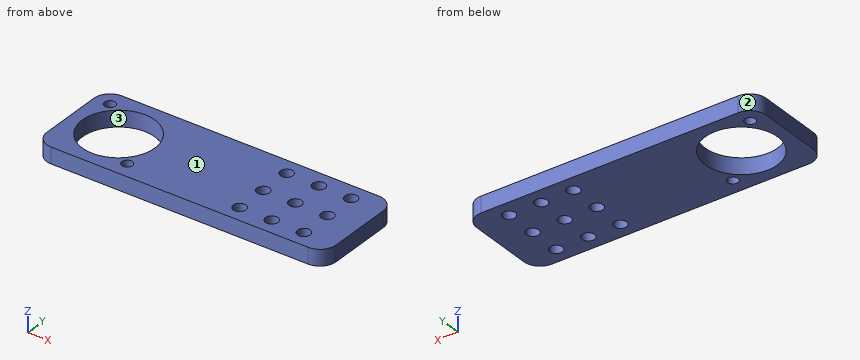
from build123d import *

# Parameters (mm, degrees)
SKETCH1_R           = 14.3002
SKETCH1_R_2         = 2.0828
SKETCH1_R_3         = 2.4892
BOSS_EXTRUDE1_DEPTH = 6.35


with BuildPart() as part:
    # Sketch1 → Boss-Extrude1 (new body)
    with BuildSketch(Plane.XY):
        with BuildLine():
            Line((114.3, -12.7), (114.3, 12.7))
            ThreePointArc((114.3, 12.7), (112.440128061, 17.190128061), (107.95, 19.05))
            Line((107.95, 19.05), (6.35, 19.05))
            ThreePointArc((6.35, 19.05), (1.859871939, 17.190128061), (0, 12.7))
            Line((0, 12.7), (0, -12.7))
            ThreePointArc((0, -12.7), (1.859871939, -17.190128061), (6.35, -19.05))
            Line((6.35, -19.05), (107.95, -19.05))
            ThreePointArc((107.95, -19.05), (112.440128061, -17.190128061), (114.3, -12.7))
        make_face()
        with Locations((19.05, 0)):
            Circle(SKETCH1_R, mode=Mode.SUBTRACT)
        with Locations((6.244154771, 12.805845229)):
            Circle(SKETCH1_R_2, mode=Mode.SUBTRACT)
        with Locations((31.75, -12.7)):
            Circle(SKETCH1_R_2, mode=Mode.SUBTRACT)
        with Locations((88.9, 12.7)):
            Circle(SKETCH1_R_3, mode=Mode.SUBTRACT)
        with Locations((101.6, 12.7)):
            Circle(SKETCH1_R_3, mode=Mode.SUBTRACT)
        with Locations((88.9, 0)):
            Circle(SKETCH1_R_3, mode=Mode.SUBTRACT)
        with Locations((101.6, 0)):
            Circle(SKETCH1_R_3, mode=Mode.SUBTRACT)
        with Locations((88.9, -12.7)):
            Circle(SKETCH1_R_3, mode=Mode.SUBTRACT)
        with Locations((76.2, 12.7)):
            Circle(SKETCH1_R_3, mode=Mode.SUBTRACT)
        with Locations((101.6, -12.7)):
            Circle(SKETCH1_R_3, mode=Mode.SUBTRACT)
        with Locations((76.2, 0)):
            Circle(SKETCH1_R_3, mode=Mode.SUBTRACT)
        with Locations((76.2, -12.7)):
            Circle(SKETCH1_R_3, mode=Mode.SUBTRACT)
    extrude(amount=-BOSS_EXTRUDE1_DEPTH)


solid = part.part
The listing builds one solid part. Answer for the finished solid, in the listing's coordinates (mm). Face numbers are marked on the shaded views. Round coordinates to 2 decimals unless told otherwise and drop trailing zeros. Write each loop counter-clockwise with the first axis right and the second up, starting at its lowest first coordinate (ties: lowest second). Pieces come first, ordered by that corner, then holes. Notation, with made-up numbers: M -20.5,70 L 25.5,70 A25 cw 25.5,102 Z; hole C 6.5,-24.75 d8. An arc over 180 degrees is marked long. Write each question's results on one line, items separated by ' | '. Start each with the question number.
Item 1: Find section D-D on z = -2. Give the number of separate pieces and of enclosed holes in the cut face, and give its area (3 significant figures).
Item 2: Find section A-A on x = 76.2. Write down the section's boundary in (y, z), and give its area (3 significant figures).
Item 3: Find section C-C on x = 18. Write down the section's boundary in (y, z), and give its area (3 significant figures).
Item 4: Find section B-B on y = -8.5. Write down the section's boundary in (x, z).
Item 5: The mould has two halves that part along X. Classify the marked faces 1, 2 and 3: +X half, -X half, draft (parallel to the pull), parting line (faces both ways), or undercut.
Item 6: Straight lines are drawn through the part: probe 1 along Y at (x, z) = (76.2, -3); probe 2 along X at (y, z) = (13, -1.5). For each, find the intervals that lie inside material, in ascending order.
Item 7: Given pin 1 Ø1 at (x, y) = (59.5, -8.5) entering from +Z; pin 2 Ø3 at (y, z) = (-14.5, -3.5) entering from +X, each flat-ended and moving along its own axis, determine where each tip first touches the part or whether it passes through.
Answer block:
1) separate pieces: 1 | enclosed holes: 12 | area: 3,480 mm²
2) outline: M -19.05,-6.35 L -15.19,-6.35 L -15.19,0 L -19.05,0 Z; M -10.21,-6.35 L -2.49,-6.35 L -2.49,0 L -10.21,0 Z; M 2.49,-6.35 L 10.21,-6.35 L 10.21,0 L 2.49,0 Z; M 15.19,-6.35 L 19.05,-6.35 L 19.05,0 L 15.19,0 Z | area: 147 mm²
3) outline: M -19.05,-6.35 L -14.26,-6.35 L -14.26,0 L -19.05,0 Z; M 14.26,-6.35 L 19.05,-6.35 L 19.05,0 L 14.26,0 Z | area: 60.8 mm²
4) outline: M 0,-6.35 L 7.55,-6.35 L 7.55,0 L 0,0 Z; M 30.55,-6.35 L 114.3,-6.35 L 114.3,0 L 30.55,0 Z
5) face 1: draft | face 2: -X half | face 3: undercut
6) probe 1: y = -19.05 to -15.19, -10.21 to -2.49, 2.49 to 10.21, 15.19 to 19.05 | probe 2: x = 0.01 to 4.17, 8.32 to 13.09, 25.01 to 73.73, 78.67 to 86.43, 91.37 to 99.13, 104.07 to 114.29
7) pin 1: stops at z = 0 | pin 2: stops at x = 114.29
